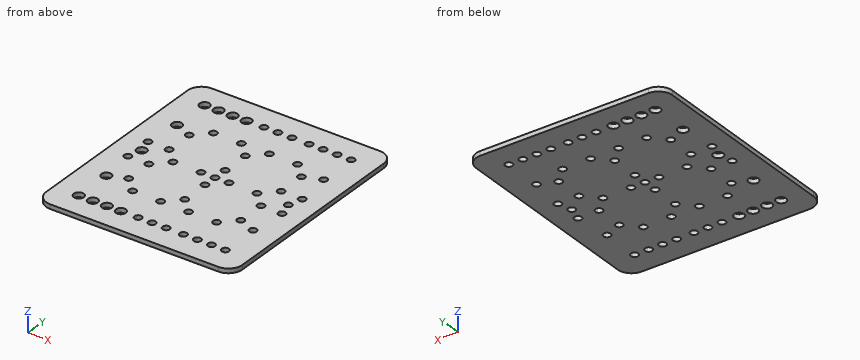
```python
from build123d import *

# Parameters (mm, degrees)
SKETCH1_W           = 140
SKETCH1_H           = 160
SKETCH1_R           = 2.6
SKETCH1_R_2         = 3.55
BOSS_EXTRUDE1_DEPTH = 3.2
FILLET1_R           = 10


with BuildPart() as part:
    # Sketch1 → Boss-Extrude1 (new body)
    with BuildSketch(Plane.XY):
        Rectangle(SKETCH1_W, SKETCH1_H)
        Circle(SKETCH1_R, mode=Mode.SUBTRACT)
        with Locations((10, 0)):
            Circle(SKETCH1_R, mode=Mode.SUBTRACT)
        with Locations((-40, 10)):
            Circle(SKETCH1_R, mode=Mode.SUBTRACT)
        with Locations((30, 0)):
            Circle(SKETCH1_R, mode=Mode.SUBTRACT)
        with Locations((-10, 0)):
            Circle(SKETCH1_R, mode=Mode.SUBTRACT)
        with Locations((40, 10)):
            Circle(SKETCH1_R, mode=Mode.SUBTRACT)
        with Locations((-30, 0)):
            Circle(SKETCH1_R, mode=Mode.SUBTRACT)
        with Locations((0, 10)):
            Circle(SKETCH1_R, mode=Mode.SUBTRACT)
        with Locations((-52.3, 35)):
            Circle(SKETCH1_R_2, mode=Mode.SUBTRACT)
        with Locations((52.3, 35)):
            Circle(SKETCH1_R, mode=Mode.SUBTRACT)
        with Locations((22.3, 62.3)):
            Circle(SKETCH1_R, mode=Mode.SUBTRACT)
        with Locations((0, 30)):
            Circle(SKETCH1_R, mode=Mode.SUBTRACT)
        with Locations((-10, 40)):
            Circle(SKETCH1_R, mode=Mode.SUBTRACT)
        with Locations((52.3, 0)):
            Circle(SKETCH1_R, mode=Mode.SUBTRACT)
        with Locations((-52.3, 0)):
            Circle(SKETCH1_R_2, mode=Mode.SUBTRACT)
        with Locations((-30, 40)):
            Circle(SKETCH1_R, mode=Mode.SUBTRACT)
        with Locations((-52.3, 62.3)):
            Circle(SKETCH1_R_2, mode=Mode.SUBTRACT)
        with Locations((-40, 30)):
            Circle(SKETCH1_R, mode=Mode.SUBTRACT)
        with Locations((40, 30)):
            Circle(SKETCH1_R, mode=Mode.SUBTRACT)
        with Locations((30, 40)):
            Circle(SKETCH1_R, mode=Mode.SUBTRACT)
        with Locations((52.3, 62.3)):
            Circle(SKETCH1_R, mode=Mode.SUBTRACT)
        with Locations((10, 40)):
            Circle(SKETCH1_R, mode=Mode.SUBTRACT)
        with Locations((-42.3, 62.3)):
            Circle(SKETCH1_R_2, mode=Mode.SUBTRACT)
        with Locations((-32.3, 62.3)):
            Circle(SKETCH1_R_2, mode=Mode.SUBTRACT)
        with Locations((-22.3, -62.3)):
            Circle(SKETCH1_R_2, mode=Mode.SUBTRACT)
        with Locations((55, -10)):
            Circle(SKETCH1_R, mode=Mode.SUBTRACT)
        with Locations((42.3, 62.3)):
            Circle(SKETCH1_R, mode=Mode.SUBTRACT)
        with Locations((-55, -10)):
            Circle(SKETCH1_R, mode=Mode.SUBTRACT)
        with Locations((-10, -62.3)):
            Circle(SKETCH1_R, mode=Mode.SUBTRACT)
        with Locations((0, 62.3)):
            Circle(SKETCH1_R, mode=Mode.SUBTRACT)
        with Locations((10, 62.3)):
            Circle(SKETCH1_R, mode=Mode.SUBTRACT)
        with Locations((-10, 62.3)):
            Circle(SKETCH1_R, mode=Mode.SUBTRACT)
        with Locations((10, -62.3)):
            Circle(SKETCH1_R, mode=Mode.SUBTRACT)
        with Locations((0, -62.3)):
            Circle(SKETCH1_R, mode=Mode.SUBTRACT)
        with Locations((32.3, -62.3)):
            Circle(SKETCH1_R, mode=Mode.SUBTRACT)
        with Locations((42.3, -62.3)):
            Circle(SKETCH1_R, mode=Mode.SUBTRACT)
        with Locations((-55, 10)):
            Circle(SKETCH1_R, mode=Mode.SUBTRACT)
        with Locations((55, 10)):
            Circle(SKETCH1_R, mode=Mode.SUBTRACT)
        with Locations((-32.3, -62.3)):
            Circle(SKETCH1_R_2, mode=Mode.SUBTRACT)
        with Locations((-42.3, -62.3)):
            Circle(SKETCH1_R_2, mode=Mode.SUBTRACT)
        with Locations((10, -40)):
            Circle(SKETCH1_R, mode=Mode.SUBTRACT)
        with Locations((52.3, -62.3)):
            Circle(SKETCH1_R, mode=Mode.SUBTRACT)
        with Locations((30, -40)):
            Circle(SKETCH1_R, mode=Mode.SUBTRACT)
        with Locations((40, -30)):
            Circle(SKETCH1_R, mode=Mode.SUBTRACT)
        with Locations((-40, -30)):
            Circle(SKETCH1_R, mode=Mode.SUBTRACT)
        with Locations((-52.3, -62.3)):
            Circle(SKETCH1_R_2, mode=Mode.SUBTRACT)
        with Locations((-30, -40)):
            Circle(SKETCH1_R, mode=Mode.SUBTRACT)
        with Locations((-10, -40)):
            Circle(SKETCH1_R, mode=Mode.SUBTRACT)
        with Locations((-22.3, 62.3)):
            Circle(SKETCH1_R_2, mode=Mode.SUBTRACT)
        with Locations((0, -30)):
            Circle(SKETCH1_R, mode=Mode.SUBTRACT)
        with Locations((32.3, 62.3)):
            Circle(SKETCH1_R, mode=Mode.SUBTRACT)
        with Locations((22.3, -62.3)):
            Circle(SKETCH1_R, mode=Mode.SUBTRACT)
        with Locations((52.3, -35)):
            Circle(SKETCH1_R, mode=Mode.SUBTRACT)
        with Locations((-52.3, -35)):
            Circle(SKETCH1_R_2, mode=Mode.SUBTRACT)
        with Locations((0, -10)):
            Circle(SKETCH1_R, mode=Mode.SUBTRACT)
        with Locations((40, -10)):
            Circle(SKETCH1_R, mode=Mode.SUBTRACT)
        with Locations((-40, -10)):
            Circle(SKETCH1_R, mode=Mode.SUBTRACT)
    extrude(amount=-BOSS_EXTRUDE1_DEPTH)

    # Fillet1
    fillet1_edges = [part.edges().sort_by_distance(p)[0] for p in [
        (70, -80, -1.6),
        (-70, -80, -1.6),
        (-70, 80, -1.6),
        (70, 80, -1.6),
    ]]
    fillet(fillet1_edges, radius=FILLET1_R)


solid = part.part
```
Verification items for the finished model (mm, model axes). Coordinates: 2 decimals unless noted, no trailing zeros. Loops run counter-clockwise (first coordinate to the right, second up) from the corner with the lowest first, then second, coordinate; pieces in that order, holes last. Notation, with made-up numbers: (26, -5) - (64, -5) arc R8 cw to (64, 10) - close; hole circle Ø6 at (-11, 79). An arc over 180 degrees is marked (long way). Return JSON: item names as keys, results as strings.
1. Section check A-A, the plane x = -10. Record the boundary of the cut face in (y, z), then the cut area to 3 significant figures.
Established:
{"outline": "(-80, -3.2) - (-64.9, -3.2) - (-64.9, 0) - (-80, 0) - close; (-59.7, -3.2) - (-42.6, -3.2) - (-42.6, 0) - (-59.7, 0) - close; (-37.4, -3.2) - (-2.6, -3.2) - (-2.6, 0) - (-37.4, 0) - close; (2.6, -3.2) - (37.4, -3.2) - (37.4, 0) - (2.6, 0) - close; (42.6, -3.2) - (59.7, -3.2) - (59.7, 0) - (42.6, 0) - close; (64.9, -3.2) - (80, -3.2) - (80, 0) - (64.9, 0) - close", "area": "429 mm2"}
2. Section check B-B, the plane y = 35. Record the boundary of the cut face in (x, z), then the cut area to 3 significant figures.
Established:
{"outline": "(-70, -3.2) - (-55.85, -3.2) - (-55.85, 0) - (-70, 0) - close; (-48.75, -3.2) - (49.7, -3.2) - (49.7, 0) - (-48.75, 0) - close; (54.9, -3.2) - (70, -3.2) - (70, 0) - (54.9, 0) - close", "area": "409 mm2"}
3. Go/stop test with a flat-tipped pin: pin 1 (7 mm diameter, centred on x = 52.3, y = -62.3, fed in from -Z). Record where the tip stops, or that it passes through.
Established:
{"pin 1": "stops at z = -3.2"}
4. Section check D-D, the plane z = -0.85. Count the separate pieces of the cut face and the enclosed holes in it, then the cut area to 3 significant figures.
Established:
{"separate pieces": "1", "enclosed holes": "57", "area": "20,900 mm2"}
5. Thickness scan on L1, parallel to Y at x = -30.5, z = -2.8; L2, parallel to Y at x = -32, z = -2; L3, parallel to Y at x = -20.5, z = -2.3. Record the ranges inside material, lowest first.
Established:
{"L1": "y = -80 to -65.36, -59.24 to -42.55, -37.45 to -2.55, 2.55 to 37.45, 42.55 to 59.24, 65.36 to 80", "L2": "y = -80 to -65.84, -58.76 to -41.66, -38.34 to -1.66, 1.66 to 38.34, 41.66 to 58.76, 65.84 to 80", "L3": "y = -80 to -65.36, -59.24 to 59.24, 65.36 to 80"}
6. Section check C-C, the plane x = 22.3. Record the boundary of the cut face in (y, z).
Established:
{"outline": "(-80, -3.2) - (-64.9, -3.2) - (-64.9, 0) - (-80, 0) - close; (-59.7, -3.2) - (59.7, -3.2) - (59.7, 0) - (-59.7, 0) - close; (64.9, -3.2) - (80, -3.2) - (80, 0) - (64.9, 0) - close"}
